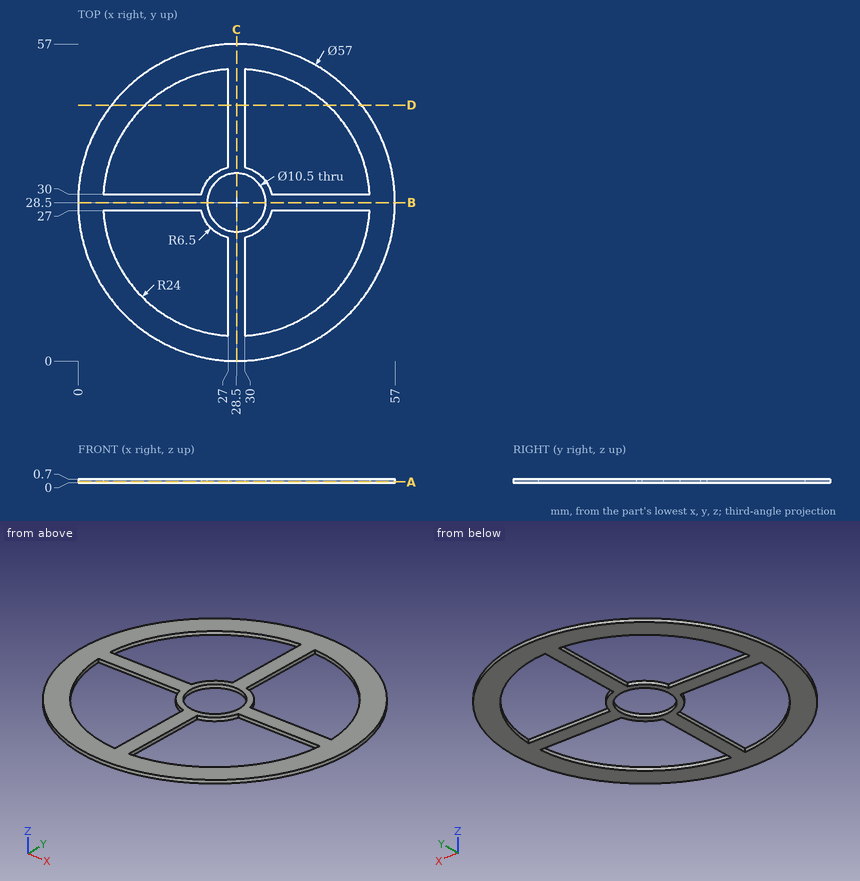
Check sheet for the drawn part. Datum: minimum x, y, z corner. Units: mm. Coordinates: 2 decimals unless noted, no trailing zeros. Order: outer loops, then holes, each group sorted by start corner. A loop starts at its lowest first (then second) coordinate and runs counter-clockwise, first axis right, second up. Notation, with made-up numbers: M 25,84 L 50,84 A24 ccw 50,98 Z; hole C 74.5,36.25 d4. An arc over 180 degrees is marked long. One line per item, written item: value. Start each with the question number.
Item 1: Scan lines: probe 1 along Y at (x, z) = (28.5, 0.15); probe 2 along X at (y, z) = (33, 0.3) (1 decimal). Record each from-to range of solid material in increasing order.
Item 2: Gauge pin test, flat end, axial feed: pin 1 (9.5 mm diameter, centred on x = 28.5, y = 28.5, fed in from +Z). Record the tip position at first contact, or that the pin passes through.
Item 3: Sectioned sample at B-B (y = 28.5). Enter the section's corners in (x, z).
Item 4: Sectioned sample at D-D (y = 46). Enter the section's corners in (x, z), then the cut area to 3 significant figures.
Item 5: Sectioned sample at A-A (z = 0.2). Count the separate pieces of the cut face and the enclosed holes in it, then the cut area to 3 significant figures.
Conclusion:
1. probe 1: y = 0 to 23.25, 33.75 to 57
1. probe 2: x = 0.4 to 4.9, 23.8 to 25.8, 31.2 to 33.2, 52.1 to 56.6
2. pin 1: passes through
3. outline: M 0,0 L 23.25,0 L 23.25,0.7 L 0,0.7 Z; M 33.75,0 L 57,0 L 57,0.7 L 33.75,0.7 Z
4. outline: M 6.01,0 L 12.08,0 L 12.08,0.7 L 6.01,0.7 Z; M 27,0 L 30,0 L 30,0.7 L 27,0.7 Z; M 44.92,0 L 50.99,0 L 50.99,0.7 L 44.92,0.7 Z
4. area: 10.6 mm^2
5. separate pieces: 1
5. enclosed holes: 5
5. area: 999 mm^2
